Design review of the part built by this model. Coordinates are the model's own, in mm. A direction names the side the tool comes from. Round coordinates to 2 decimals unless told otherwise and drop trailing zeros. Loops run counter-clockwise (first coordinate to the right, second up) from the corner with the lowest first, then second, coordinate; pieces in that order, holes last. Notation, with made-up numbers: (-14, 13.5) - (36, 13.5) arc R30 cw to (36, 42.5) - close; hole circle Ø6 at (17, 9.5). An arc over 180 degrees is marked (long way). Answer as CSV lines item,"result". Start each with the question number.
(1) Consider section C-C (z = -34.5). Give the boundary of the cut face in (x, y).
(2) Consider section D-D (x = -61). Give the boundary of the cut face in (y, z).
(3) Consider section B-B (x = -53.5). Give the boundary of the cut face in (y, z), and give its area (3 significant figures).
(4) For faces 5 (the flat face through (-19.151, -6, 12)), 6 (the cylindrical face through (-54.114, -1.288, 43.918)), list the 3-axis set-ups (+Z, -Z, +X, -X, +Y, -Y) from which the entire face can be reached by the end or side of a thin tool; tool diameter is ignored.
(5) For P1, Ø7.5, axis at x = -25.05, z = 66.66, coming from the -Y side; P2, Ø2, axis at x = -49, z = 29, coming from the -Y side; P3, Ø5, axis at x = -52.5, y = -5.5, coming from the +Z side, all flat-tipped, find the tip position at first contact; note any pin that passes through.
(6) Mouldability with a two-part tool opening along Z and no side actions: class faces 1 (the flat face through (-18, -8.966, 31)), 2 (the cylindrical face through (-18.138, -4.546, -48.053)), 3 (the cylindrical face through (-18.05, -4.55, 73.24)), 4 (the cylindrical face through (-72.526, -5.798, 71.641)) as released by +Z, released by -Z, zero draft, split by the parting line, or undercut.
(7) Consider section A-A (y = -3.75). Give the boundary of the cut face in (x, z).
(8) Wall thickness on L1, parallel to X at y = -7.75, z = -33.5; L2, parallel to Z at x = -28, y = -2.75; L3, parallel to Z at x = -25, y = -8.5: over which ranges is each line inside the solid? List them lowest first.
from build123d import *

# Parameters (mm, degrees)
F1_DEPTH = 8.9662
F2_R     = 5.08
F3_R     = 5.08
F4_R     = 3.1670818849
F5_DEPTH = 25.4
F6_R     = 10.0620941007
F7_DEPTH = 25.4
F8_T     = -2.54


with BuildPart() as f1:
    # F0 (on Front) → F1 (new body)
    with BuildSketch(Plane.XZ):
        Polygon((-75.792866245, 74.9588643271), (-75.792866245, -49.5011356729), (-16.610866245, -49.5011356729), (-16.610866245, 74.7600470389), align=None)
    extrude(amount=F1_DEPTH)

    # F2
    f2_edges = [f1.edges().sort_by_distance(p)[0] for p in [
        (-16.610866, -4.4831, 74.760047),
        (-16.610866, -4.4831, -49.501136),
    ]]
    fillet(f2_edges, radius=F2_R)

    # F3
    f3_edges = [f1.edges().sort_by_distance(p)[0] for p in [
        (-75.792866, -4.4831, 74.958864),
        (-75.792866, -4.4831, -49.501136),
    ]]
    fillet(f3_edges, radius=F3_R)

    # F4 (on face) → F5 (cut)
    with BuildSketch(Plane.XZ.offset(8.9662)):
        with Locations((-25.0480864197, 66.6592344642)):
            Circle(F4_R)
    extrude(amount=-F5_DEPTH, mode=Mode.SUBTRACT)

    # F6 (on face) → F7 (cut)
    with BuildSketch(Plane.XZ.offset(8.9662)):
        with Locations((-46.6981939971, 37.1179692447)):
            Circle(F6_R)
    extrude(amount=-F7_DEPTH, mode=Mode.SUBTRACT)

    # F8
    f8_openings = [f1.faces().sort_by_distance(p)[0] for p in [
        (-46.282621, -8.9662, 11.323406),
        (-56.760288, -4.4831, 37.117969),
        (-28.215168, -4.4831, 66.659234),
    ]]
    offset(amount=F8_T, openings=f8_openings)


solid = f1.part
Determined:
1,outline,"(-75.79, -8.97) - (-73.25, -8.97) - (-73.25, -2.54) - (-19.15, -2.54) - (-19.15, -8.97) - (-16.61, -8.97) - (-16.61, 0) - (-75.79, 0) - close"
2,outline,"(-8.97, -49.5) - (0, -49.5) - (0, 74.91) - (-8.97, 74.91) - (-8.97, 72.37) - (-2.54, 72.37) - (-2.54, -46.96) - (-8.97, -46.96) - close"
3,outline,"(-8.97, -49.5) - (0, -49.5) - (0, 29.7) - (-2.54, 29.7) - (-2.54, -46.96) - (-8.97, -46.96) - close; (-8.97, 72.34) - (-2.54, 72.34) - (-2.54, 44.53) - (0, 44.53) - (0, 74.88) - (-8.97, 74.88) - close"
3,area,"311 mm^2"
4,face 5,"-Y"
4,face 6,"+Y, -Y"
5,P1,"stops at y = -2.54"
5,P2,"passes through"
5,P3,"stops at z = 74.89"
6,face 1,"zero draft"
6,face 2,"released by -Z"
6,face 3,"released by +Z"
6,face 4,"undercut"
7,outline,"(-75.79, -44.42) arc R5.08 ccw to (-70.71, -49.5) - (-21.69, -49.5) arc R5.08 ccw to (-16.61, -44.42) - (-16.61, 69.7) arc R5.08 ccw to (-21.67, 74.78) - (-70.7, 74.94) arc R5.08 ccw to (-75.79, 69.86) - close; hole (-73.25, -44.42) arc R2.54 ccw to (-70.71, -46.96) - (-21.69, -46.96) arc R2.54 ccw to (-19.15, -44.42) - (-19.15, 69.7) arc R2.54 ccw to (-21.68, 72.24) - (-70.7, 72.4) arc R2.54 ccw to (-73.25, 69.86) - close"
8,L1,"x = -75.79 to -73.25, -19.15 to -16.61"
8,L2,"z = -49.5 to -46.96, 72.26 to 74.8"
8,L3,"z = -49.5 to -46.96, 72.25 to 74.79"
